Geometry: final body of the model. Coordinates: model frame, mm. Give positions to 0.01 mm unless a question says otherwise; leave off trailing zeros. Loops run counter-clockwise (first coordinate to the right, second up) from the corner with the lowest first, then second, coordinate; pieces in that order, holes last. Notation, with made-up numbers: (-1.5, 47) -> (26.5, 47) arc R15 cw to (26.5, 76) -> close; hole circle Ø4 at (78, 61). An arc over 180 degrees is marked (long way). Answer in a Markdown table with one row per item. Add a question column.
from build123d import *

# Parameters (mm, degrees)
F0_W     = 43.18
F0_H     = 33.02
F1_DEPTH = 17.78
F2_R     = 15.24
F3_R     = 15.24
F4_R     = 8.89


with BuildPart() as f1:
    # F0 (on Front) → F1 (new body, symmetric)
    with BuildSketch(Plane.XZ):
        Rectangle(F0_W, F0_H)
    extrude(amount=F1_DEPTH, both=True)

    # F2
    f2_edges = [f1.edges().sort_by_distance(p)[0] for p in [
        (0, -17.78, 16.51),
    ]]
    fillet(f2_edges, radius=F2_R)

    # F3
    f3_edges = [f1.edges().sort_by_distance(p)[0] for p in [
        (0, -17.78, -16.51),
        (0, 17.78, -16.51),
        (0, 17.78, 16.51),
    ]]
    fillet(f3_edges, radius=F3_R)

    # F4
    f4_edges = [f1.edges().sort_by_distance(p)[0] for p in [
        (21.59, -13.316307, 12.046307),
        (-21.59, -13.316307, -12.046307),
    ]]
    fillet(f4_edges, radius=F4_R)


solid = f1.part
(1) Cut plane B-B on x = -10.5. Return the cut outline in (y, z).
(2) Cut plane A-A on z = 0. Return the cut outline in (x, y).
(3) Material intervals for line 1 along X through (y, z) = (-2, 8); line 2 along Z through (x, y) = (13, 2.5); line 3 along X through (y, z) = (-14, -9.5), sorted ascending. Write a range as from..to.
(4) Pin query (flat end, axial travel): pin 1 Ø1 at (y, z) = (-4, 11) entering from -X; pin 2 Ø1.5 at (x, z) = (16.5, 6.5) entering from -Y; pin 3 Ø1.5 at (x, z) = (14.5, -5.5) entering from -Y. Return the tip coordinate at first contact, or that it passes through.
Answer list:
| question | item | result |
|---|---|---|
| 1 | outline | (-17.78, -1.27) arc R15.24 ccw to (-2.54, -16.51) -> (2.54, -16.51) arc R15.24 ccw to (17.78, -1.27) -> (17.78, 1.27) arc R15.24 ccw to (2.54, 16.51) -> (-2.54, 16.51) arc R15.24 ccw to (-17.78, 1.27) -> close |
| 2 | outline | (-21.59, -8.89) arc R8.89 ccw to (-12.7, -17.78) -> (12.7, -17.78) arc R8.89 ccw to (21.59, -8.89) -> (21.59, 8.89) arc R8.89 ccw to (12.7, 17.78) -> (-12.7, 17.78) arc R8.89 ccw to (-21.59, 8.89) -> close |
| 3 | line 1 | x = -21.58..21.58 |
| 3 | line 2 | z = -16.5..16.5 |
| 3 | line 3 | x = -17.04..17.04 |
| 4 | pin 1 | stops at x = -21.07 |
| 4 | pin 2 | stops at y = -16.38 |
| 4 | pin 3 | stops at y = -17.24 |
